Work out the finished part from the listing and answer in its coordinate system (mm). A direction names the side the tool comes from. Give positions to 0.01 mm unless a question says otherwise; leave off trailing zeros. Loops run counter-clockwise (first coordinate to the right, second up) from the corner with the lowest first, then second, coordinate; pieces in that order, holes last. Notation, with made-up numbers: M 28.25,56.5 L 73.25,56.5 A27 ccw 73.25,78.5 Z; hole C 20.5,-38 d8. An arc over 180 degrees is marked long. Write item = value, one per line. Start each with the question number.
1. Consider L1, parallel to Z at x = -9, y = 11.5; L2, parallel to X at y = 0.95, z = -14.92; L3, parallel to Y at x = -17.5, z = 20.5. Determine where each line is inside the solid, lowest interval first. Write a range as [from, to].
2. Section D-D on z = 56 is taken. Determine the outline of the cut face in (x, y), plus the area to 3 significant figures.
3. The mould has two halves that part along X. Classify faces 1 (the face through (-103.19, 0.986, -39.764)), 2 (the face through (93.3, 1, -39.9)), 3 (the face through (6, 9, 91.5)): released by +X, released by -X, zero draft, split by the parting line, or undercut.
4. Flat-ended cylindrical pins translate along their axes: pin 1 Ø9 at (x, z) = (-121, 38.5) entering from +Y; pin 2 Ø3 at (y, z) = (11, -0.5) entering from -X; pin 3 Ø1 at (x, y) = (74.5, 1) entering from +Z. Find the tip coordinate at first contact, or state that the pin passes through.
5. For faces 4 (the face through (131.2, 1.5, 32.5)), 5 (the face through (-103.544, 0.986, 39.969)), 6 (the face through (164, 9, 0)), determine the directions among +Z, -Z, +X, -X, +Y, -Y from which every point of the face is accessible in a straight line to the end or side of a thin tool.
6. Section B-B on y = 8 is taken. Determine the outline of the cut face in (x, z), plus the area to 3 significant figures.
7. Section C-C on x = -2 is taken. Determine the outline of the cut face in (y, z), plus the area to 3 significant figures.
8. Section A-A on x = -121 is taken. Determine the outline of the cut face in (y, z).
```python
from build123d import *

# Parameters (mm, degrees)
SKETCH1_R           = 4
SKETCH1_R_2         = 2
SKETCH1_R_3         = 2.5
BOSS_EXTRUDE1_DEPTH = 2
SKETCH2_W           = 1
SKETCH2_H           = 65
BOSS_EXTRUDE2_DEPTH = 12
FILLET1_R           = 2.5


with BuildPart() as part:
    # Sketch1 → Boss-Extrude1 (new body)
    with BuildSketch(Plane(origin=(0, 0, 0), x_dir=(1, 0, 0), z_dir=(0, 1, 0))):
        with BuildLine():
            Line((165, -32.5), (165, 32.5))
            Line((165, 32.5), (97, 32.5))
            Line((97, 32.5), (89.5, 47.5))
            Line((89.5, 47.5), (57.5, 47.5))
            Line((57.5, 47.5), (57.5, 59.5))
            Line((57.5, 59.5), (83.5, 59.5))
            Line((83.5, 59.5), (67, 92.5))
            Line((67, 92.5), (-56.134697257, 92.5))
            Line((-56.134697257, 92.5), (-90.733708845, 32.572754038))
            Line((-90.733708845, 32.572754038), (-116, 47.160254038))
            ThreePointArc((-116, 47.160254038), (-121, 48.5), (-126, 47.160254038))
            Line((-126, 47.160254038), (-165, 24.643593539))
            Line((-165, 24.643593539), (-165, -24.643593539))
            Line((-165, -24.643593539), (-126, -47.160254038))
            ThreePointArc((-126, -47.160254038), (-121, -48.5), (-116, -47.160254038))
            Line((-116, -47.160254038), (-90.733708845, -32.572754038))
            Line((-90.733708845, -32.572754038), (-56.134697257, -92.5))
            Line((-56.134697257, -92.5), (67, -92.5))
            Line((67, -92.5), (97, -32.5))
            Line((97, -32.5), (165, -32.5))
        make_face()
        with Locations(Location((-121, -38.5, 0), (0, 0, 270))):
            Circle(SKETCH1_R, mode=Mode.SUBTRACT)
        with Locations(Location((-160.497563939, -14.92, 0), (0, 0, 270))):
            Circle(SKETCH1_R_2, mode=Mode.SUBTRACT)
        with Locations(Location((103, -16.25, 0), (0, 0, 270))):
            Circle(SKETCH1_R_3, mode=Mode.SUBTRACT)
        with Locations(Location((153, -16.25, 0), (0, 0, 270))):
            Circle(SKETCH1_R_3, mode=Mode.SUBTRACT)
        with Locations(Location((-160.497578586, 14.92, 0), (0, 0, 270))):
            Circle(SKETCH1_R_2, mode=Mode.SUBTRACT)
        with Locations(Location((-121, 38.5, 0), (0, 0, 270))):
            Circle(SKETCH1_R, mode=Mode.SUBTRACT)
        with Locations(Location((103, 16.25, 0), (0, 0, 270))):
            Circle(SKETCH1_R_3, mode=Mode.SUBTRACT)
        with Locations(Location((153, 16.25, 0), (0, 0, 270))):
            Circle(SKETCH1_R_3, mode=Mode.SUBTRACT)
    extrude(amount=BOSS_EXTRUDE1_DEPTH)

    # Sketch2 → Boss-Extrude2 (add)
    with BuildSketch(Plane(origin=(0, 2, 0), x_dir=(1, 0, 0), z_dir=(0, 1, 0))):
        Polygon((-56.134697257, -92.5), (67, -92.5), (67.5, -91.5), (-56.712047526, -91.5), align=None)
        Polygon((-56.134697257, 92.5), (67, 92.5), (67.5, 91.5), (-56.712047526, 91.5), align=None)
        with Locations((164.5, 0)):
            Rectangle(SKETCH2_W, SKETCH2_H)
    extrude(amount=BOSS_EXTRUDE2_DEPTH)

    # Fillet1
    # the kernel refuses this fillet: 2.5 mm, written as the material it adds along each edge
    with BuildSketch(Plane(origin=(73.75, 2, -91.5), x_dir=(0, 1, 0), z_dir=(-1, 0, 0))) as fillet1_piece_1_section:
        with BuildLine():
            CenterArc((FILLET1_R, -FILLET1_R), FILLET1_R, 90, 90)
            Line((0, -FILLET1_R), (0, 0))
            Line((0, 0), (FILLET1_R, 0))
        make_face()
    fillet1_piece_1 = extrude(amount=136.712047526, mode=Mode.PRIVATE)
    fillet1_piece_1 = split(fillet1_piece_1, bisect_by=Plane(origin=(-41.43720377, 2.56450665, -117.956805463), z_dir=(0.8660254037844399, 0, 0.49999999999999795)), keep=Keep.TOP, mode=Mode.PRIVATE)
    fillet1_piece_1 = split(fillet1_piece_1, bisect_by=Plane(origin=(55.3017959, 2.56450665, -115.8964082), z_dir=(-0.894427190999916, 0, 0.447213595499958)), keep=Keep.TOP, mode=Mode.PRIVATE)
    add(fillet1_piece_1)
    with BuildSketch(Plane(origin=(164, 2, 32.5), x_dir=(0, 1, 0), z_dir=(0, 0, -1))) as fillet1_piece_2:
        with BuildLine():
            CenterArc((FILLET1_R, -FILLET1_R), FILLET1_R, 90, 90)
            Line((0, -FILLET1_R), (0, 0))
            Line((0, 0), (FILLET1_R, 0))
        make_face()
    extrude(amount=65)
    with BuildSketch(Plane(origin=(73.75, 2, 91.5), x_dir=(0, 0, -1), z_dir=(-1, 0, 0))) as fillet1_piece_3_section:
        with BuildLine():
            CenterArc((FILLET1_R, -FILLET1_R), FILLET1_R, 90, 90)
            Line((0, -FILLET1_R), (0, 0))
            Line((0, 0), (FILLET1_R, 0))
        make_face()
    fillet1_piece_3 = extrude(amount=136.712047526, mode=Mode.PRIVATE)
    fillet1_piece_3 = split(fillet1_piece_3, bisect_by=Plane(origin=(55.3017959, 2.56450665, 115.8964082), z_dir=(-0.894427190999916, 0, -0.44721359549995787)), keep=Keep.TOP, mode=Mode.PRIVATE)
    fillet1_piece_3 = split(fillet1_piece_3, bisect_by=Plane(origin=(-41.43720377, 2.56450665, 117.956805463), z_dir=(0.8660254037844399, 0, -0.49999999999999795)), keep=Keep.TOP, mode=Mode.PRIVATE)
    add(fillet1_piece_3)
    # the kernel refuses this fillet: 2.5 mm, written as the material it takes off along each edge
    with BuildSketch(Plane(origin=(-59.837047526, 14, -86.087341226), x_dir=(0, -1, 0), z_dir=(0.5000000000000019, 0, -0.8660254037844376)), Plane(origin=(-59.837047526, 14, 86.087341226), x_dir=(0.8660254037844394, 0, -0.49999999999999867), z_dir=(0.4999999999999987, 0, 0.8660254037844395))) as fillet1_2_piece_1:
        with BuildLine():
            CenterArc((FILLET1_R, -FILLET1_R), FILLET1_R, 90, 90)
            Line((0, -FILLET1_R), (0, 0))
            Line((0, 0), (FILLET1_R, 0))
        make_face()
    extrude(amount=13.654700538, mode=Mode.SUBTRACT)
    with BuildSketch(Plane(origin=(64.204915028, 14, -98.090169944), x_dir=(0, -1, 0), z_dir=(0.447213595499958, 0, 0.894427190999916))) as fillet1_2_piece_2:
        with BuildLine():
            CenterArc((FILLET1_R, -FILLET1_R), FILLET1_R, 90, 90)
            Line((0, -FILLET1_R), (0, 0))
            Line((0, 0), (FILLET1_R, 0))
        make_face()
    extrude(amount=13.618033989, mode=Mode.SUBTRACT)
    with BuildSketch(Plane(origin=(157.75, 14, -32.5), x_dir=(0, -1, 0), z_dir=(1, 0, 0)), Plane(origin=(171.25, 14, 32.5), x_dir=(0, -1, 0), z_dir=(-1, 0, 0))) as fillet1_2_piece_3:
        with BuildLine():
            CenterArc((FILLET1_R, -FILLET1_R), FILLET1_R, 90, 90)
            Line((0, -FILLET1_R), (0, 0))
            Line((0, 0), (FILLET1_R, 0))
        make_face()
    extrude(amount=13.5, mode=Mode.SUBTRACT)
    with BuildSketch(Plane(origin=(73.25, 0, -92.5), x_dir=(0, 0, 1), z_dir=(-1, 0, 0))) as fillet1_2_piece_4:
        with BuildLine():
            CenterArc((FILLET1_R, FILLET1_R), FILLET1_R, 180, 90)
            Line((0, FILLET1_R), (0, 0))
            Line((0, 0), (FILLET1_R, 0))
        make_face()
    extrude(amount=135.634697257, mode=Mode.SUBTRACT)
    with BuildSketch(Plane(origin=(165, 0, 38.75), x_dir=(-1, 0, 0), z_dir=(0, 0, -1))) as fillet1_2_piece_5:
        with BuildLine():
            CenterArc((FILLET1_R, FILLET1_R), FILLET1_R, 180, 90)
            Line((0, FILLET1_R), (0, 0))
            Line((0, 0), (FILLET1_R, 0))
        make_face()
    extrude(amount=77.5, mode=Mode.SUBTRACT)
    with BuildSketch(Plane(origin=(-62.384697257, 0, 92.5), x_dir=(0, 1, 0), z_dir=(1, 0, 0))) as fillet1_2_piece_6:
        with BuildLine():
            CenterArc((FILLET1_R, -FILLET1_R), FILLET1_R, 90, 90)
            Line((0, -FILLET1_R), (0, 0))
            Line((0, 0), (FILLET1_R, 0))
        make_face()
    extrude(amount=135.634697257, mode=Mode.SUBTRACT)
    with BuildSketch(Plane(origin=(64.204915028, 14, 98.090169944), x_dir=(0, -1, 0), z_dir=(0.447213595499958, 0, -0.894427190999916))) as fillet1_2_piece_7:
        with BuildLine():
            CenterArc((FILLET1_R, FILLET1_R), FILLET1_R, 180, 90)
            Line((0, FILLET1_R), (0, 0))
            Line((0, 0), (FILLET1_R, 0))
        make_face()
    extrude(amount=13.618033989, mode=Mode.SUBTRACT)


solid = part.part
```
Verdict:
q1.L1 = [-92.5, -91.5], [91.5, 92.5]
q1.L2 = [-165, -162.5], [-158.5, 100.88], [105.12, 150.88], [155.12, 164.46]
q1.L3 = [0, 2]
q2.outline = M -77.21,0 L 85.25,0 L 85.25,2 L -77.21,2 Z
q2.area = 325 mm2
q3.face_1 = undercut
q3.face_2 = released by +X
q3.face_3 = zero draft
q4.pin_1 = 2
q4.pin_2 = 164
q4.pin_3 = 78.5
q5.face_4 = +Z, +X, +Y, -Y
q5.face_5 = +Z, +Y, -Y
q5.face_6 = +Z, -Z, -X, +Y
q6.outline = M -56.71,-91.5 L -56.13,-92.5 L 67,-92.5 L 67.5,-91.5 Z; M -56.71,91.5 L 67.5,91.5 L 67,92.5 L -56.13,92.5 Z; M 164,-32.5 L 165,-32.5 L 165,32.5 L 164,32.5 Z
q6.area = 312 mm2
q7.outline = M 0,-90 A2.5 ccw 2.5,-92.5 L 14,-92.5 L 14,-91.5 L 4.5,-91.5 A2.5 cw 2,-89 L 2,89 A2.5 cw 4.5,91.5 L 14,91.5 L 14,92.5 L 2.5,92.5 A2.5 ccw 0,90 Z
q7.area = 394 mm2
q8.outline = M 0,-48.5 L 2,-48.5 L 2,-42.5 L 0,-42.5 Z; M 0,-34.5 L 2,-34.5 L 2,34.5 L 0,34.5 Z; M 0,42.5 L 2,42.5 L 2,48.5 L 0,48.5 Z
